Can you work these out from the model? Positions are in its coordinate system, mm. A direction names the side the tool comes from. Give positions to 0.01 mm unless a question says otherwise; leave off trailing zeros. Loops run counter-clockwise (first coordinate to the right, second up) from the corner with the lowest first, then second, coordinate; pieces in that order, holes last. Notation, with made-up numbers: M 24.5,-2 L 43.5,-2 A12 ccw 43.5,2 Z; hole C -40,-8 d7. An arc over 180 degrees is marked long. Answer as a JSON object with one key per item and string values.
```python
from build123d import *

# Parameters (mm, degrees)
F0_W     = 750
F0_H     = 1932
F0_W_2   = 550
F0_H_2   = 100
F1_DEPTH = 25
F3_R     = 6
F4_DEPTH = 4


with BuildPart() as f1:
    # F0 (on Front) → F1 (new body, symmetric)
    with BuildSketch(Plane.XZ):
        Rectangle(F0_W, F0_H)
        Polygon((-275, -366), (-275, 866), (275, 866), (275, -366), (275, -466), (275, -866), (-275, -866), (-275, -466), align=None, mode=Mode.SUBTRACT)
        with Locations((0, -416)):
            Rectangle(F0_W_2, F0_H_2)
    extrude(amount=F1_DEPTH, both=True)

    # F3 (on offset) → F4 (join)
    with BuildSketch(Plane.YZ.offset(-375)):
        with Locations((10, 766)):
            Circle(F3_R)
        with Locations((10, -766)):
            Circle(F3_R)
    extrude(amount=-F4_DEPTH)


solid = f1.part
```
1) Please list where these lines run through material, in increasing order: line 1 along Z through (x, y) = (90.5, 17); line 2 along X through (y, z) = (11, 399). Write a range as from..to.
Answer list:
{"line 1": "-966..-866, -466..-366, 866..966", "line 2": "-375..-275, 275..375"}
2) If we mould it in two halves opening along X, with no side actions, what happens to faces 3 (the flat face through (-275, 0, -669)), 4 (the flat face through (-375, 0, -14)), 5 (the flat face through (-339, 25, 14))? For each: +X half, -X half, draft (parallel to the pull), parting line (faces both ways), or undercut.
Answer list:
{"face 3": "undercut", "face 4": "-X half", "face 5": "draft"}
3) Suppose I cut it at A-A, the plane x = 189. Write out the boundary of the cut face in (y, z), and give its area (3 significant figures).
Answer list:
{"outline": "M -25,-966 L 25,-966 L 25,-866 L -25,-866 Z; M -25,-466 L 25,-466 L 25,-366 L -25,-366 Z; M -25,866 L 25,866 L 25,966 L -25,966 Z", "area": "15,000 mm^2"}
4) Suppose I cut it at C-C, the plane z = 679. Write out the boundary of the cut face in (x, y), and give its area (3 significant figures).
Answer list:
{"outline": "M -375,-25 L -275,-25 L -275,25 L -375,25 Z; M 275,-25 L 375,-25 L 375,25 L 275,25 Z", "area": "10,000 mm^2"}
5) For faces 1 (the flat face through (-339, -25, 14)), 2 (the flat face through (275, 0, -663)), which set-ups out of +Z, -Z, +X, -X, +Y, -Y let a thin tool reach every point of the face, with its end or its side?
Answer list:
{"face 1": "+Z, -Z, +X, -X, -Y", "face 2": "+Y, -Y"}
6) Suppose I cut it at B-B, the plane y = -8. Write out the boundary of the cut face in (x, z), and give its area (3 significant figures).
Answer list:
{"outline": "M -375,-966 L 375,-966 L 375,966 L -375,966 Z; hole M -275,-866 L 275,-866 L 275,-466 L -275,-466 Z; hole M -275,-366 L 275,-366 L 275,866 L -275,866 Z", "area": "551,000 mm^2"}
